from build123d import *

# Parameters (mm, degrees)
F0_W      = 32.5
F0_H      = 3
F1_DEPTH  = 80
F3_DEPTH  = 4
F4_W      = 17.5
F4_H      = 3
F5_DEPTH  = 25
F6_SIZE   = 15
F7_SIZE   = 5
F8_W      = 62.9999996811
F8_H      = 9.7999996811
F9_DEPTH  = 4
F10_SIZE  = 3
F11_SIZE  = 5
F12_W     = 25
F12_H     = 25
F13_DEPTH = 5
F15_DEPTH = 25


with BuildPart() as f1:
    # F0 (on Top) → F1 (new body)
    with BuildSketch(Plane.XY):
        Polygon((-35.5, 0), (-32.5, 0), (-32.5, 3), (-32.5, 14.8), (-35.5, 14.8), align=None)
        Polygon((32.5, 3), (32.5, 0), (35.5, 0), (35.5, 14.8), (32.5, 14.8), align=None)
        with Locations((-16.25, 1.5)):
            Rectangle(F0_W, F0_H)
        with Locations((16.25, 1.5)):
            Rectangle(F0_W, F0_H)
        Polygon((-35.5, 14.8), (-32.5, 14.8), (-27.5, 14.8), (-27.5, 17.8), (-35.5, 17.8), align=None)
        Polygon((27.5, 14.8), (32.5, 14.8), (35.5, 14.8), (35.5, 17.8), (27.5, 17.8), align=None)
    extrude(amount=F1_DEPTH)

    # F2 (on face) → F3 (join)
    with BuildSketch(Plane.XY.offset(80)):
        Polygon((27.5, 17.8), (-27.5, 17.8), (-27.5, 14.8), (-32.5, 14.8), (-32.5, 3), (32.5, 3), (32.5, 14.8), (27.5, 14.8), align=None)
        Polygon((-27.5, 17.8), (-35.5, 17.8), (-35.5, 0), (35.5, 0), (35.5, 17.8), (27.5, 17.8), (27.5, 14.8), (32.5, 14.8), (32.5, 3), (-32.5, 3), (-32.5, 14.8), (-27.5, 14.8), align=None)
    extrude(amount=F3_DEPTH)

    # F4 (on face) → F5 (join)
    with BuildSketch(Plane(origin=(0, 0, 80), x_dir=(1, 0, 0), z_dir=(0, 0, -1))):
        with Locations((-18.75, -16.3)):
            Rectangle(F4_W, F4_H)
        with Locations((18.75, -16.3)):
            Rectangle(F4_W, F4_H)
    extrude(amount=F5_DEPTH)

    # F6
    f6_edges = [f1.edges().sort_by_distance(p)[0] for p in [
        (-10, 16.3, 55),
        (10, 16.3, 55),
    ]]
    chamfer(f6_edges, length=F6_SIZE)

    # F7
    f7_edges = [f1.edges().sort_by_distance(p)[0] for p in [
        (-10, 16.3, 70),
        (10, 16.3, 70),
    ]]
    chamfer(f7_edges, length=F7_SIZE)

    # F8 (on face) → F9 (cut)
    with BuildSketch(Plane.XY.offset(84)):
        with Locations((0, 8.9)):
            Rectangle(F8_W, F8_H)
    extrude(amount=-F9_DEPTH, mode=Mode.SUBTRACT)

    # F10
    f10_edges = [f1.edges().sort_by_distance(p)[0] for p in [
        (-31.5, 13.8, 82),
        (-31.5, 4, 82),
        (31.5, 4, 82),
        (31.5, 13.8, 82),
        (10, 16.3, 80),
        (-10, 16.3, 80),
    ]]
    chamfer(f10_edges, length=F10_SIZE)

    # F11
    f11_edges = [f1.edges().sort_by_distance(p)[0] for p in [
        (-27.5, 16.3, 0),
        (27.5, 16.3, 0),
    ]]
    chamfer(f11_edges, length=F11_SIZE)

    # F12 (on face) → F13 (join)
    with BuildSketch(Plane.XZ):
        with Locations((0, 38.6652871966)):
            Rectangle(F12_W, F12_H)
    extrude(amount=F13_DEPTH)

    # F14 (on face) → F15 (cut)
    with BuildSketch(Plane.XY.offset(51.1652871966)):
        Polygon((8.5, 0), (-8.5, 0), (-3.5, -5), (3.5, -5), align=None)
    extrude(amount=-F15_DEPTH, mode=Mode.SUBTRACT)


solid = f1.part
Geometry: final body of the model. Coordinates: model frame, mm. A direction names the side the tool comes from. Coordinates: 2 decimals unless noted, no trailing zeros. Order: outer loops, then holes, each group sorted by start corner. A loop starts at its lowest first (then second) coordinate and runs counter-clockwise, first axis right, second up.
1) Section D-D (z = 56.5). Return loops of the section in (x, y).
Result sheet:
outline: (-35.5, 0) - (35.5, 0) - (35.5, 17.8) - (23.5, 17.8) - (23.5, 14.8) - (32.5, 14.8) - (32.5, 3) - (-32.5, 3) - (-32.5, 14.8) - (-23.5, 14.8) - (-23.5, 17.8) - (-35.5, 17.8) - close
2) First-contact query: P1, Ø7.5, axis at x = 18, z = 21, coming from the -Y side; P2, Ø8, axis at x = -17.5, z = 10, coming from the +Y side; P3, Ø3, axis at x = 25.5, y = 17, coming from the -Z side; P4, Ø2, axis at y = -1.5, z = 75.5, coming from the +X side. Flat tips, straight axial feed; report the tip coordinate or a pass-through.
Result sheet:
P1: stops at y = 0
P2: stops at y = 3
P3: stops at z = 55
P4: passes through
3) Section A-A (x = 21). Return loops of the section in (y, z).
Result sheet:
outline: (0, 0) - (3, 0) - (3, 80) - (4, 80) - (4, 84) - (0, 84) - close; (13.8, 80) - (14.8, 80) - (14.8, 59) - (17.8, 59) - (17.8, 84) - (13.8, 84) - close
4) Ray query, probe 1 along X at (y, z) = (9.5, 9); probe 2 along Y at (x, z) = (-18.5, 67); probe 3 along X at (y, z) = (16.25, 26). Return the intervals inside material, ascending.
Result sheet:
probe 1: x = -35.5 to -32.5, 32.5 to 35.5
probe 2: y = 0 to 3, 14.8 to 17.8
probe 3: x = -35.5 to -27.5, 27.5 to 35.5
5) Set-up query: faces 1 (the flat face through (-8, -5, 39)), 2 (the flat face through (-27.5, 16, 30)), 3 (the flat face through (0, 3, 39)), 4 (the flat face through (15, 17.8, 71)), 5 (the flat face through (-30, 12.3, 82)). Return all of +Z, -Z, +X, -X, +Y, -Y with unobstructed straight access to the full face (end or side cutting, diameter ignored); none if empty.
Result sheet:
face 1: +Z, -Z, +X, -X, -Y
face 2: -Z, +Y
face 3: -Z
face 4: +Z, -Z, +X, -X, +Y
face 5: +Z, -Z
6) Draft query along X for faces 6 (the flat face through (-9, -3, 26.165)), 7 (the flat face through (11.793, 16.321, 70.672)), 8 (the flat face through (12.5, -2, 38)). Return one class per face: released by +X, released by -X, zero draft, split by the parting line, or undercut.
Result sheet:
face 6: zero draft
face 7: undercut
face 8: released by +X
7) Section C-C (x = 4.5). Return loops of the section in (y, z), then the cut area to 3 significant figures.
Result sheet:
outline: (-5, 26.17) - (-4, 26.17) - (-4, 51.17) - (-5, 51.17) - close; (0, 0) - (3, 0) - (3, 80) - (4, 80) - (4, 84) - (0, 84) - close; (13.8, 80) - (17.8, 80) - (17.8, 84) - (13.8, 84) - close
area: 297 mm2
8) Section B-B (y = 8.25). Return loops of the section in (x, z), then the cut area to 3 significant figures.
Result sheet:
outline: (-35.5, 0) - (-32.5, 0) - (-32.5, 80) - (-31.5, 80) - (-31.5, 84) - (-35.5, 84) - close; (31.5, 80) - (32.5, 80) - (32.5, 0) - (35.5, 0) - (35.5, 84) - (31.5, 84) - close
area: 512 mm2
